Build history of the part. All positions in model axes, mm. A direction names the side the tool comes from. Give positions to 0.01 mm unless a question says otherwise; leave off trailing zeros. Loops run counter-clockwise (first coordinate to the right, second up) from the corner with the lowest first, then second, coordinate; pieces in that order, holes last.
1) Wall check: line 1 (Y direction, x = 27.5, z = 6); line 2 (Y direction, x = 27, z = 5.25); line 3 (X direction, y = 17.5, z = 5.5). Give the ranges that are in metal, low to high.
2) Band-saw the part on A-A on y = 45. List the corners of the cut face in (x, z).
3) Flat gauge pins, fed straight in: P1, Ø10, axis at x = -25, y = 29, coming from the +Z side; P2, Ø4, axis at y = -10.5, z = 2, coming from the -X side; P3, Ø24, axis at x = 31.5, y = -32.5, coming from the -Z side; P4, Ø1, axis at y = -4.5, z = 3.5, coming from the -X side. Where does each tip first touch, or does it go through?
4) Band-saw the part on C-C on y = -31. List the corners of the cut face in (x, z).
5) 3-axis set-ups, long thin cutter, end or side, ignore diameter. For faces 1 (the flat face through (24, -24, 5)), 2 (the flat face through (-21.83, 26.87, 2.46)), 3 (the flat face through (-26.65, 21.61, 2.46)), 4 (the cylindrical face through (0.22, 13.325, 2.535)): which of +Z, -Z, +X, -X, +Y, -Y reach the whole face in a straight line?
6) Band-saw the part on D-D on x = 26. List the corners of the cut face in (y, z).
7) Band-saw the part on B-B on x = 41. List the corners of the cut face in (y, z), then the cut area to 3 significant figures.
```python
from build123d import *

# Parameters (mm, degrees)
BOSS_EXTRUDE1_DEPTH = 5
FILLET1_R           = 20
SKETCH3_R           = 24
SKETCH3_R_2         = 22
BOSS_EXTRUDE2_DEPTH = 2


with BuildPart() as part:
    # Sketch2 → Boss-Extrude1 (new body)
    with BuildSketch(Plane.XY):
        Polygon((0, 5.039474274), (29.300068016, 34.339542291), (34.339542291, 29.300068016), (5.039474274, 0), (34.339542291, -29.300068016), (29.300068016, -34.339542291), (0, -5.039474274), (-29.300068016, -34.339542291), (-34.339542291, -29.300068016), (-5.039474274, 0), (-34.339542291, 29.300068016), (-29.300068016, 34.339542291), align=None)
    extrude(amount=BOSS_EXTRUDE1_DEPTH)

    # Fillet1
    fillet1_edges = [part.edges().sort_by_distance(p)[0] for p in [
        (0, -5.039474274, 2.5),
        (-5.039474274, 0, 2.5),
        (0, 5.039474274, 2.5),
        (5.039474274, 0, 2.5),
    ]]
    fillet(fillet1_edges, radius=FILLET1_R)

    # Sketch3 → Boss-Extrude2 (add)
    # profile 1 of 4: a face of its own
    with BuildSketch(Plane.XY.offset(5)):
        with Locations(Location((-31.819805153, 31.819805153, 0), (0, 0, 306.147120123))):
            Circle(SKETCH3_R)
        with Locations(Location((-31.819805153, 31.819805153, 0), (0, 0, 305.673554169))):
            Circle(SKETCH3_R_2, mode=Mode.SUBTRACT)
    # profile 2 of 4: a face of its own
    with BuildSketch(Plane.XY.offset(5)):
        with Locations(Location((31.819805153, 31.819805153, 0), (0, 0, 216.147120123))):
            Circle(SKETCH3_R)
        with Locations(Location((31.819805153, 31.819805153, 0), (0, 0, 215.673554169))):
            Circle(SKETCH3_R_2, mode=Mode.SUBTRACT)
    # profile 3 of 4: a face of its own
    with BuildSketch(Plane.XY.offset(5)):
        with Locations(Location((31.819805153, -31.819805153, 0), (0, 0, 143.852879877))):
            Circle(SKETCH3_R)
        with Locations(Location((31.819805153, -31.819805153, 0), (0, 0, 144.326445831))):
            Circle(SKETCH3_R_2, mode=Mode.SUBTRACT)
    # profile 4 of 4: a face of its own
    with BuildSketch(Plane.XY.offset(5)):
        with Locations(Location((-31.819805153, -31.819805153, 0), (0, 0, 53.852879877))):
            Circle(SKETCH3_R)
        with Locations(Location((-31.819805153, -31.819805153, 0), (0, 0, 54.326445831))):
            Circle(SKETCH3_R_2, mode=Mode.SUBTRACT)
    extrude(amount=BOSS_EXTRUDE2_DEPTH)


solid = part.part
```
Findings below:
1. line 1: y = -55.43 to -53.39, -10.25 to -8.21, 8.21 to 10.25, 53.39 to 55.43
1. line 2: y = -55.33 to -53.29, -10.35 to -8.31, 8.31 to 10.35, 53.29 to 55.33
1. line 3: x = -51.08 to -48.52, -15.12 to -12.56, 12.56 to 15.12, 48.52 to 51.08
2. outline: (-51.88, 5) - (-49.43, 5) - (-49.43, 7) - (-51.88, 7) - close; (-14.2, 5) - (-11.76, 5) - (-11.76, 7) - (-14.2, 7) - close; (11.76, 5) - (14.2, 5) - (14.2, 7) - (11.76, 7) - close; (49.43, 5) - (51.88, 5) - (51.88, 7) - (49.43, 7) - close
3. P1: stops at z = 5
3. P2: stops at x = -17.71
3. P3: stops at z = 0
3. P4: stops at x = -13.96
4. outline: (-55.81, 5) - (-53.8, 5) - (-53.8, 7) - (-55.81, 7) - close; (-32.64, 0) - (-25.96, 0) - (-25.96, 5) - (-32.64, 5) - close; (-9.84, 5) - (-7.83, 5) - (-7.83, 7) - (-9.84, 7) - close; (7.83, 5) - (9.84, 5) - (9.84, 7) - (7.83, 7) - close; (25.96, 0) - (32.64, 0) - (32.64, 5) - (25.96, 5) - close; (53.8, 5) - (55.81, 5) - (55.81, 7) - (53.8, 7) - close
5. face 1: +Z
5. face 2: +Z, -Z, +Y
5. face 3: +Z, -Z, -X
5. face 4: -Z, +Y
6. outline: (-55.1, 5) - (-53.04, 5) - (-53.04, 7) - (-55.1, 7) - close; (-31.04, 0) - (-20.96, 0) - (-20.96, 5) - (-31.04, 5) - close; (-10.6, 5) - (-8.54, 5) - (-8.54, 7) - (-10.6, 7) - close; (8.54, 5) - (10.6, 5) - (10.6, 7) - (8.54, 7) - close; (20.96, 0) - (31.04, 0) - (31.04, 5) - (20.96, 5) - close; (53.04, 5) - (55.1, 5) - (55.1, 7) - (53.04, 7) - close
7. outline: (-53.99, 5) - (-51.81, 5) - (-51.81, 7) - (-53.99, 7) - close; (-11.83, 5) - (-9.64, 5) - (-9.64, 7) - (-11.83, 7) - close; (9.64, 5) - (11.83, 5) - (11.83, 7) - (9.64, 7) - close; (51.81, 5) - (53.99, 5) - (53.99, 7) - (51.81, 7) - close
7. area: 17.5 mm2
